from build123d import *

# Parameters (mm, degrees)
SKETCH1_W           = 22
SKETCH1_H           = 9.5
BOSS_EXTRUDE1_DEPTH = 12
CUT_EXTRUDE1_REACH  = 20.848
SKETCH2_W           = 21
SKETCH2_H           = 1.851123708


with BuildPart() as part:
    # Sketch1 → Boss-Extrude1 (new body)
    with BuildSketch(Plane(origin=(0, 0, 0), x_dir=(1, 0, 0), z_dir=(0, 1, 0))):
        Rectangle(SKETCH1_W, SKETCH1_H)
    extrude(amount=BOSS_EXTRUDE1_DEPTH)

    # Sketch2 → Cut-Extrude1 (cut, up to next)
    with BuildSketch(Plane.XY.offset(4.75), mode=Mode.PRIVATE) as cut_extrude1_sk1:
        with Locations((0, -0.425561854)):
            Rectangle(SKETCH2_W, SKETCH2_H)
    cut_extrude1_tool1 = extrude(cut_extrude1_sk1.sketch, amount=-CUT_EXTRUDE1_REACH, mode=Mode.PRIVATE) & part.part
    add(cut_extrude1_tool1.solids().sort_by_distance((0, -0.425562, 4.75))[0], mode=Mode.SUBTRACT)


solid = part.part
Model file for the job. Use its own axes, mm. Give positions to 0.01 mm unless a question says otherwise; leave off trailing zeros. Order: outer loops, then holes, each group sorted by start corner. A loop starts at its lowest first (then second) coordinate and runs counter-clockwise, first axis right, second up. Notation, with made-up numbers: (44, -30) - (77, -30) arc R8 ccw to (77, -15) - close; hole circle Ø7 at (42.5, 56.5). An arc over 180 degrees is marked (long way). One line per item, written item: value.
Item 1: Pin check, flat tip, straight feed: pin 1 Ø3 at (x, z) = (-5, -1) entering from -Y. Stop position of the tip, or through.
Response values:
pin 1: y = 0.5
Item 2: Slice it at A-A (z = 1). List the corners of the cut face in (x, y).
Response values:
outline: (-11, 0) - (-10.5, 0) - (-10.5, 0.5) - (10.5, 0.5) - (10.5, 0) - (11, 0) - (11, 12) - (-11, 12) - close
Item 3: Slice it at B-B (x = -8.5). List the corners of the cut face in (y, z), then the cut area to 3 significant figures.
Response values:
outline: (0.5, -4.75) - (12, -4.75) - (12, 4.75) - (0.5, 4.75) - close
area: 109 mm2
Item 4: Two-plate mould, pull along X, no slides. Class faces 1 (the flat face through (0, 0.5, 0)), 2 (the flat face through (11, 6, 0)), 3 (the flat face through (-11, 6, 0)): released by +X, released by -X, zero draft, split by the parting line, or undercut.
Response values:
face 1: undercut
face 2: released by +X
face 3: released by -X
Item 5: Wall check: line 1 (Y direction, x = 9.25, z = 0.5). Give the ranges that are in metal, low to high.
Response values:
line 1: 0.5 to 12
